```python
from build123d import *

# Parameters (mm, degrees)
BOSS_EXTRUDE1_DEPTH = 42
SKETCH2_R           = 12
SKETCH2_R_2         = 1.5
CUT_EXTRUDE1_DEPTH  = 5
SKETCH3_R           = 2
CUT_EXTRUDE2_DEPTH  = 5
CHAMFER2_SIZE       = 1
FILLET1_R           = 4


with BuildPart() as part:
    # Sketch1 → Boss-Extrude1 (new body)
    with BuildSketch(Plane(origin=(0, 0, 0), x_dir=(1, 0, 0), z_dir=(0, 1, 0))):
        Polygon((0, 0), (0, 51), (-20, 51), (-20, 55), (4, 55), (4, 0), align=None)
    extrude(amount=BOSS_EXTRUDE1_DEPTH)

    # Sketch2 → Cut-Extrude1 (cut, through all)
    with BuildSketch(Plane.ZY):
        with Locations((-21, 21)):
            Circle(SKETCH2_R)
        with Locations((-36.5, 36.5)):
            Circle(SKETCH2_R_2)
        with Locations((-5.5, 36.5)):
            Circle(SKETCH2_R_2)
        with Locations((-5.5, 5.5)):
            Circle(SKETCH2_R_2)
        with Locations((-36.5, 5.5)):
            Circle(SKETCH2_R_2)
    extrude(amount=-CUT_EXTRUDE1_DEPTH, mode=Mode.SUBTRACT)

    # Sketch3 → Cut-Extrude2 (cut, through all)
    with BuildSketch(Plane.XY.offset(-51)):
        with Locations((-10, 32)):
            Circle(SKETCH3_R)
        with Locations((-10, 10)):
            Circle(SKETCH3_R)
    extrude(amount=-CUT_EXTRUDE2_DEPTH, mode=Mode.SUBTRACT)

    # Chamfer2
    chamfer2_edges = [part.edges().sort_by_distance(p)[0] for p in [
        (0, 21, -33),
    ]]
    chamfer(chamfer2_edges, length=CHAMFER2_SIZE)

    # Fillet1
    fillet1_edges = [part.edges().sort_by_distance(p)[0] for p in [
        (4, 21, -55),
        (-20, 42, -53),
        (2, 42, 0),
        (-20, 0, -53),
        (2, 0, 0),
    ]]
    fillet(fillet1_edges, radius=FILLET1_R)


solid = part.part
```
Input: part model. Units: mm. Frame: model coordinates. A direction names the side the tool comes from. Coordinates: 2 decimals unless noted, no trailing zeros. Order: outer loops, then holes, each group sorted by start corner. A loop starts at its lowest first (then second) coordinate and runs counter-clockwise, first axis right, second up. Notation, with made-up numbers: (9, -18) - (33, -18) arc R19 ccw to (33, -4) - close; hole circle Ø7 at (34.5, 45.25). An arc over 180 degrees is marked (long way). Return JSON: item names as keys, results as strings.
Q1. Cut plane A-A (x = -10). Return loops of the section in (y, z).
The answers:
{"outline": "(0, -55) - (8, -55) - (8, -51) - (0, -51) - close; (12, -55) - (30, -55) - (30, -51) - (12, -51) - close; (34, -55) - (42, -55) - (42, -51) - (34, -51) - close"}
Q2. Ray query, probe 1 along Y at (x, z) = (2.2, -5.5); probe 2 along Y at (x, z) = (2.85, -21); probe 3 along Y at (x, z) = (-10, -52.2). Return the intervals inside material, ascending.
The answers:
{"probe 1": "y = 0 to 4, 7 to 35, 38 to 42", "probe 2": "y = 0 to 9, 33 to 42", "probe 3": "y = 0 to 8, 12 to 30, 34 to 42"}
Q3. Cut plane C-C (z = -21). Return loops of the section in (x, y), then the cut area to 3 significant figures.
The answers:
{"outline": "(0, 0) - (4, 0) - (4, 9) - (1, 9) - (0, 8) - close; (0, 34) - (1, 33) - (4, 33) - (4, 42) - (0, 42) - close", "area": "71.0 mm2"}
Q4. Access query for faces 4 (the flat face through (-10, 21, -51)), 5 (the cylindrical face through (-18.797, 40.859, -53.028)). Directions: +Z, -Z, +X, -X, +Y, -Y. A direction counts if a zero-diameter tool reaches every point of the face in a straight line with its end or side. Return the directions, or none.
The answers:
{"face 4": "+Z, -X, +Y, -Y", "face 5": "+Z, -Z, -X, +Y"}
Q5. Cut plane B-B (y = 21). Return loops of the section in (x, z).
The answers:
{"outline": "(-20, -55) - (0, -55) arc R4 ccw to (4, -51) - (4, -33) - (1, -33) - (0, -34) - (0, -51) - (-20, -51) - close; (0, -8) - (1, -9) - (4, -9) - (4, 0) - (0, 0) - close"}
Q6. Cut plane D-D (y = 36.5). Return loops of the section in (x, z).
The answers:
{"outline": "(-20, -55) - (0, -55) arc R4 ccw to (4, -51) - (4, -38) - (0, -38) - (0, -51) - (-20, -51) - close; (0, -35) - (4, -35) - (4, -7) - (0, -7) - close; (0, -4) - (4, -4) - (4, 0) - (0, 0) - close"}
Q7. First-contact query: pin 1 (4 mm diameter, centred on x = -11, y = 6.5, fed in from +Z); pin 2 (12 mm diameter, centred on y = 5, z = -34, fed in from -X). Flat tips, straight axial feed; report the tip coordinate or a pass-through.
The answers:
{"pin 1": "stops at z = -51", "pin 2": "stops at x = 0"}
Q8. Draft query along Z for faces 1 (the cylindrical face through (1.972, 35.036, -5.825)), 2 (the flat face through (1, 42, -35)), 3 (the flat face through (2, 21, 0)). Return one class per face: +Z half, -Z half, draft (parallel to the pull), parting line (faces both ways), or undercut.
The answers:
{"face 1": "undercut", "face 2": "draft", "face 3": "+Z half"}
